Source: CAD feature listing. Evaluate the final solid. Frame: model axes, mm. Coordinates: 2 decimals unless noted, no trailing zeros. Loops run counter-clockwise (first coordinate to the right, second up) from the corner with the lowest first, then second, coordinate; pieces in that order, holes last.
from build123d import *

# Parameters (mm, degrees)
SKETCH1_R           = 177.8
BOSS_EXTRUDE1_DEPTH = 5.9944
SKETCH3_R           = 1.905
SKETCH3_W           = 5.9944
SKETCH3_H           = 25.4
SKETCH3_W_2         = 38.1
SKETCH3_H_2         = 127
SKETCH3_W_3         = 25.4
SKETCH3_H_3         = 5.9944
CUT_EXTRUDE1_DEPTH  = 5.9944


with BuildPart() as part:
    # Sketch1 → Boss-Extrude1 (new body)
    with BuildSketch(Plane.XY):
        with Locations(Location((0, 0, 0), (0, 0, 180))):
            Circle(SKETCH1_R)
    extrude(amount=BOSS_EXTRUDE1_DEPTH)

    # Sketch3 → Cut-Extrude1 (cut)
    with BuildSketch(Plane.XY.offset(5.9944)):
        with Locations((-154.4828, 25.4)):
            Circle(SKETCH3_R)
        with Locations((-154.4828, -25.4)):
            Circle(SKETCH3_R)
        with Locations((-86.8172, -25.4)):
            Circle(SKETCH3_R)
        with Locations((-86.8172, 25.4)):
            Circle(SKETCH3_R)
        with Locations((86.8172, -25.4)):
            Circle(SKETCH3_R)
        with Locations((154.4828, -25.4)):
            Circle(SKETCH3_R)
        with Locations((86.8172, 25.4)):
            Circle(SKETCH3_R)
        with Locations((154.4828, 25.4)):
            Circle(SKETCH3_R)
        with Locations((-25.4, -154.4828)):
            Circle(SKETCH3_R)
        with Locations((25.4, -154.4828)):
            Circle(SKETCH3_R)
        with Locations((-154.4828, -50.8)):
            Rectangle(SKETCH3_W, SKETCH3_H)
        with Locations((-120.65, 0)):
            Rectangle(SKETCH3_W_2, SKETCH3_H_2)
        with Locations((-154.4828, 50.8)):
            Rectangle(SKETCH3_W, SKETCH3_H)
        with Locations((-154.4828, 0)):
            Rectangle(SKETCH3_W, SKETCH3_H)
        with Locations((154.4828, 0)):
            Rectangle(SKETCH3_W, SKETCH3_H)
        with Locations((154.4828, -50.8)):
            Rectangle(SKETCH3_W, SKETCH3_H)
        with Locations((154.4828, 50.8)):
            Rectangle(SKETCH3_W, SKETCH3_H)
        with Locations((120.65, 0)):
            Rectangle(SKETCH3_W_2, SKETCH3_H_2)
        with Locations((-86.8172, 0)):
            Rectangle(SKETCH3_W, SKETCH3_H)
        with Locations((-86.8172, -50.8)):
            Rectangle(SKETCH3_W, SKETCH3_H)
        with Locations((-86.8172, 50.8)):
            Rectangle(SKETCH3_W, SKETCH3_H)
        with Locations((86.8172, -50.8)):
            Rectangle(SKETCH3_W, SKETCH3_H)
        with Locations((86.8172, 50.8)):
            Rectangle(SKETCH3_W, SKETCH3_H)
        with Locations((86.8172, 0)):
            Rectangle(SKETCH3_W, SKETCH3_H)
        with Locations((50.8, -154.4828)):
            Rectangle(SKETCH3_W_3, SKETCH3_H_3)
        with Locations((-50.8, -154.4828)):
            Rectangle(SKETCH3_W_3, SKETCH3_H_3)
        with Locations((0, -154.4828)):
            Rectangle(SKETCH3_W_3, SKETCH3_H_3)
    extrude(amount=-CUT_EXTRUDE1_DEPTH, mode=Mode.SUBTRACT)


solid = part.part
Q1. Section B-B, the plane y = 0. Return the cut outline in (x, z), plus the area to 3 significant figures.
Q2. Section D-D, the plane y = 79. Return the cut outline in (x, z), plus the area to 3 significant figures.
Q3. Line query: line 1 along X through (y, z) = (-37, 4.1); line 2 along X through (y, z) = (-154.5, 2.3); line 3 along Y through (x, z) = (113, 3.05). Output: solid intervals per line, ascending.
Q4. Section A-A, the plane x = 0. Return the cut outline in (y, z).
Q5. Contact query for flat-ended pins moving along their axis: pin 1 Ø1.8 at (x, z) = (-48.5, 3.5) entering from +Y; pin 2 Ø1 at (x, z) = (-53, 2) entering from +Y; pin 3 Ø1.8 at (y, z) = (-55, 3.5) entering from +X. Output: stop coordinate, or through.
Q6. Section C-C, the plane x = 123.5. Return the cut outline in (y, z), plus the area to 3 significant figures.
Derived:
1. outline: (-177.8, 0) - (-157.48, 0) - (-157.48, 5.99) - (-177.8, 5.99) - close; (-151.49, 0) - (-139.7, 0) - (-139.7, 5.99) - (-151.49, 5.99) - close; (-101.6, 0) - (-89.81, 0) - (-89.81, 5.99) - (-101.6, 5.99) - close; (-83.82, 0) - (83.82, 0) - (83.82, 5.99) - (-83.82, 5.99) - close; (89.81, 0) - (101.6, 0) - (101.6, 5.99) - (89.81, 5.99) - close; (139.7, 0) - (151.49, 0) - (151.49, 5.99) - (139.7, 5.99) - close; (157.48, 0) - (177.8, 0) - (177.8, 5.99) - (157.48, 5.99) - close
1. area: 1,530 mm2
2. outline: (-159.29, 0) - (159.29, 0) - (159.29, 5.99) - (-159.29, 5.99) - close
2. area: 1,910 mm2
3. line 1: x = -173.91 to -139.7, -101.6 to 101.6, 139.7 to 173.91
3. line 2: x = -87.99 to -63.5, -38.1 to -27.3, -23.5 to -12.7, 12.7 to 23.5, 27.3 to 38.1, 63.5 to 87.99
3. line 3: y = -137.27 to -63.5, 63.5 to 137.27
4. outline: (-177.8, 0) - (-157.48, 0) - (-157.48, 5.99) - (-177.8, 5.99) - close; (-151.49, 0) - (177.8, 0) - (177.8, 5.99) - (-151.49, 5.99) - close
5. pin 1: stops at y = 171.31
5. pin 2: stops at y = 169.87
5. pin 3: stops at x = 169.37
6. outline: (-127.91, 0) - (-63.5, 0) - (-63.5, 5.99) - (-127.91, 5.99) - close; (63.5, 0) - (127.91, 0) - (127.91, 5.99) - (63.5, 5.99) - close
6. area: 772 mm2
